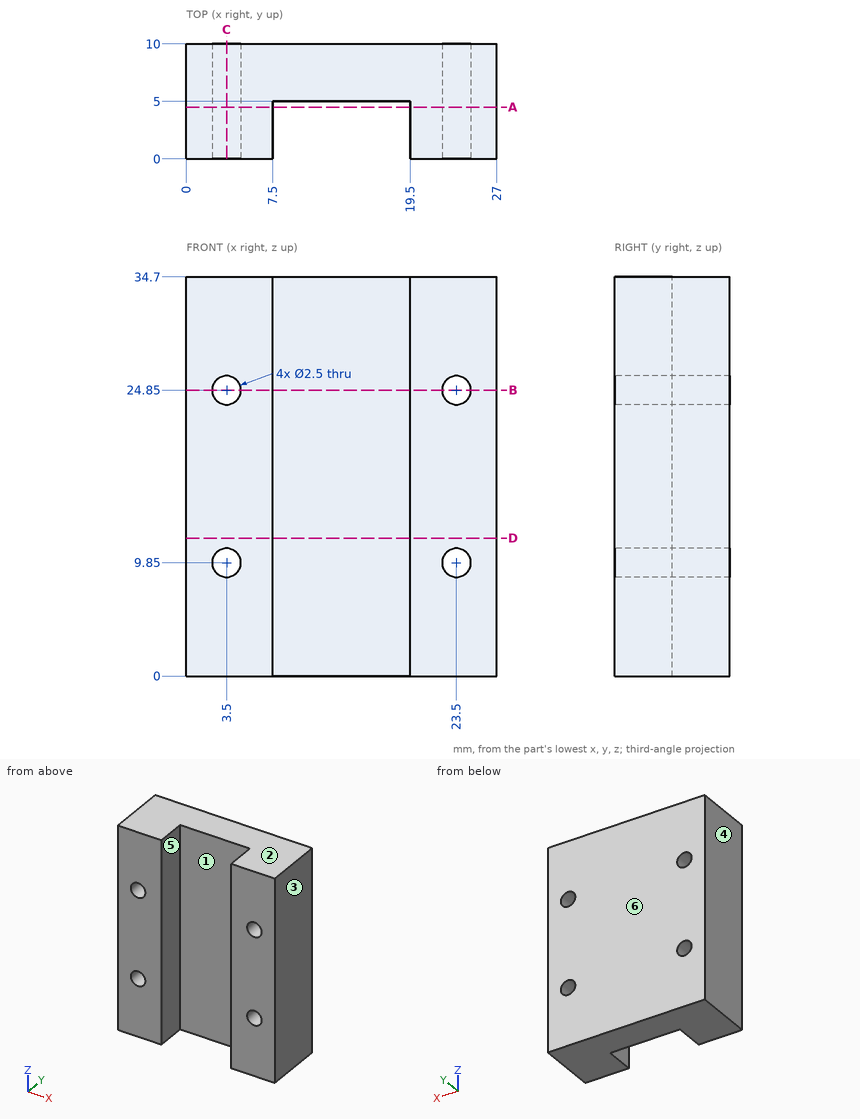
Study the drawing (mm; zero at the part's minimum x, y, z) and answer. A direction names the side the tool comes from. Round coordinates to 2 decimals unless told otherwise and drop trailing zeros. Loops run counter-clockwise (first coordinate to the right, second up) from the corner with the lowest first, then second, coordinate; pieces in that order, holes last. Notation, with made-up numbers: (74.5, 11.25) - (132.5, 11.25) arc R24 ccw to (132.5, 50.25) - close; hole circle Ø9 at (60, -5). An arc over 180 degrees is marked (long way). Use one line per item in the form item = value. Start each with the question number.
1. The part is cut by section C-C on x = 3.5. Determine the outline of the cut face in (y, z), then the cut area to 3 significant figures.
2. For a pull along X with two mould halves and no side action, classify the marked faces 1, 2, 3 and 4 as pulls with the +X half, pulls with the -X half, needs draft (parallel to the pull), parting line crosses it, or undercut.
3. Given pin 1 Ø2.5 at (y, z) = (3.5, 23) entering from -X; pin 2 Ø6 at (x, z) = (12.5, 26) entering from -Y, each flat-ended and moving along its own axis, determine where each tip first touches the part or whether it passes through.
4. A tool of negligible diameter and unlimited length cuts with its end or side. For the marked faces 5 and 6, from which of +Z, -Z, +X, -X, +Y, -Y can it reach the whole face along a straight path? Write none if from no direction.
5. Consider line 1 (X direction, y = 3, z = 24.85); line 2 (Z direction, x = 23.5, y = 7.75); line 3 (X direction, y = 7.25, z = 24.85). Determine where each line is inside the solid, lowest interval first. Write a range as [from, to].
6. The part is cut by section D-D on z = 12. Determine the outline of the cut face in (x, y).
7. The part is cut by section B-B on z = 24.85. Determine the outline of the cut face in (x, y), then the cut area to 3 significant figures.
8. The part is cut by section A-A on y = 4.5. Determine the outline of the cut face in (x, z).
Geometry check:
q1.outline = (0, 0) - (10, 0) - (10, 8.6) - (0, 8.6) - close; (0, 11.1) - (10, 11.1) - (10, 23.6) - (0, 23.6) - close; (0, 26.1) - (10, 26.1) - (10, 34.7) - (0, 34.7) - close
q1.area = 297 mm^2
q2.face_1 = undercut
q2.face_2 = needs draft
q2.face_3 = pulls with the +X half
q2.face_4 = pulls with the -X half
q3.pin_1 = 0
q3.pin_2 = 5
q4.face_5 = +Z, -Z, -Y
q4.face_6 = +Z, -Z, +X, -X, +Y
q5.line_1 = [0, 2.25], [4.75, 7.5], [19.5, 22.25], [24.75, 27]
q5.line_2 = [0, 8.6], [11.1, 23.6], [26.1, 34.7]
q5.line_3 = [0, 2.25], [4.75, 22.25], [24.75, 27]
q6.outline = (0, 0) - (7.5, 0) - (7.5, 5) - (19.5, 5) - (19.5, 0) - (27, 0) - (27, 10) - (0, 10) - close
q7.outline = (0, 0) - (2.25, 0) - (2.25, 10) - (0, 10) - close; (4.75, 0) - (7.5, 0) - (7.5, 5) - (19.5, 5) - (19.5, 0) - (22.25, 0) - (22.25, 10) - (4.75, 10) - close; (24.75, 0) - (27, 0) - (27, 10) - (24.75, 10) - close
q7.area = 160 mm^2
q8.outline = (0, 0) - (7.5, 0) - (7.5, 34.7) - (0, 34.7) - close; (19.5, 0) - (27, 0) - (27, 34.7) - (19.5, 34.7) - close; hole circle Ø2.5 at (3.5, 9.85); hole circle Ø2.5 at (3.5, 24.85); hole circle Ø2.5 at (23.5, 9.85); hole circle Ø2.5 at (23.5, 24.85)
